The model under review builds one solid part; all positions refer to its coordinate system, in mm. A direction names the side the tool comes from. Give positions to 0.01 mm unless a question says otherwise; leave off trailing zeros. Loops run counter-clockwise (first coordinate to the right, second up) from the corner with the lowest first, then second, coordinate; pieces in that order, holes last. Notation, with made-up numbers: M -40,56.5 L 5,56.5 A15 ccw 5,77.5 Z; hole C 47,31.5 d1. An arc over 180 degrees is marked long. Return JSON: item names as keys, results as strings. Group by question number.
```python
from build123d import *

# Parameters (mm, degrees)
AUFSATZ_LINEAR_AUSTRAGEN1_DEPTH = 18
AUFSATZ_LINEAR_AUSTRAGEN2_DEPTH = 2
SCHNITT_LINEAR_AUSTRAGEN1_REACH = 31.142
SCHNITT_LINEAR_AUSTRAGEN2_REACH = 35.939
SKIZZE5_W                       = 12
SKIZZE5_H                       = 15
SKIZZE7_R                       = 1.22999984
AUFSATZ_LINEAR_AUSTRAGEN3_DEPTH = 6.5
SKIZZE8_R                       = 4.22999984
SKIZZE8_R_2                     = 2.3
AUFSATZ_LINEAR_AUSTRAGEN4_DEPTH = 3
SKIZZE9_W                       = 16.252283896
SKIZZE9_H                       = 8
SKIZZE9_W_2                     = 16.225392475
AUFSATZ_LINEAR_AUSTRAGEN7_DEPTH = 3
SCHNITT_LINEAR_AUSTRAGEN3_REACH = 3.5
SKIZZE11_W                      = 10
SKIZZE11_H                      = 10
SCHNITT_LINEAR_AUSTRAGEN4_REACH = 24.734
SKIZZE13_W                      = 10
SKIZZE13_H                      = 10
SCHNITT_LINEAR_AUSTRAGEN5_REACH = 24.815
SKIZZE14_W                      = 10
SKIZZE14_H                      = 10
SCHNITT_LINEAR_AUSTRAGEN6_REACH = 3.5
SKIZZE15_W                      = 10
SKIZZE15_H                      = 10
SCHNITT_LINEAR_AUSTRAGEN7_REACH = 24.918
SKIZZE16_W                      = 10
SKIZZE16_H                      = 10
SCHNITT_LINEAR_AUSTRAGEN8_REACH = 24.774
SKIZZE17_W                      = 10
SKIZZE17_H                      = 10
SKIZZE18_W                      = 10
SKIZZE18_H                      = 1.5
SCHNITT_LINEAR_AUSTRAGEN9_DEPTH = 8


with BuildPart() as part:
    # Skizze1 → Aufsatz-Linear austragen1 (new body)
    with BuildSketch(Plane.XY):
        Polygon((-22.149859894, 27.765281808), (-11.635793215, 33.83000044), (-10.65000108, 33.83000044), (-10.65000108, 70.94999986), (10.5900012, 70.94999986), (10.5900012, 33.83000044), (11.612735063, 33.83000044), (21.946878227, 27.90320319), (54.822266278, 46.860690996), (65.431940836, 28.488460753), (35.875483821, 11.41999954), (37.79000014, 11.41999954), (37.79000014, -11.66999904), (36.372671479, -11.66999904), (65.402118422, -28.428154068), (54.791716349, -46.801638497), (21.961456264, -27.849347945), (11.636228403, -33.81000048), (10.608764603, -33.81000048), (10.588764643, -70.99999976), (-10.63000112, -70.99999976), (-10.63000112, -33.81000048), (-11.635211495, -33.81000048), (-21.94526311, -27.869445957), (-54.832668225, -46.841377939), (-65.441180026, -28.458395245), (-33.1799992, -9.82193495), (-33.1799992, 9.582671858), (-65.619428736, 28.349034811), (-55.023633975, 46.732102334), align=None)
        Polygon((-22.149950537, 26.033576659), (-11.234189479, 32.33000044), (-9.15000108, 32.33000044), (-9.15000108, 69.44999986), (9.0900012, 69.44999986), (9.0900012, 32.33000044), (11.2131258, 32.33000044), (21.948913697, 26.172853479), (54.272963006, 44.812413555), (63.382848908, 29.03729054), (31.311020441, 10.516235735), (31.653238716, 9.91999954), (36.29000014, 9.91999954), (36.29000014, -10.16999904), (31.252050971, -10.16999904), (31.132619329, -10.37701429), (63.352910716, -28.977183946), (54.242770108, -44.752743199), (21.961450411, -26.11734559), (11.234340849, -32.31000048), (9.109571053, -32.31000048), (9.089571093, -69.49999976), (-9.13000112, -69.49999976), (-9.13000112, -32.31000048), (-11.233987142, -32.31000048), (-21.945708018, -26.138007916), (-54.2831028, -44.792652518), (-63.392584266, -29.007267794), (-31.162137007, -10.388561496), (-31.6799992, -9.546253935), (-31.6799992, 9.963511331), (-31.471105622, 10.326986156), (-63.571974887, 28.897490395), (-54.473438465, 44.682904625), align=None, mode=Mode.SUBTRACT)
    extrude(amount=AUFSATZ_LINEAR_AUSTRAGEN1_DEPTH)

    # Skizze3 → Aufsatz-Linear austragen2 (add)
    with BuildSketch(Plane(origin=(0, 0, 0), x_dir=(-1, 0, 0), z_dir=(0, 0, -1))):
        Polygon((55.023633975, 46.732102334), (22.149859894, 27.765281808), (11.635793215, 33.83000044), (10.65000108, 33.83000044), (10.65000108, 70.94999986), (-10.5900012, 70.94999986), (-10.5900012, 33.83000044), (-11.612735063, 33.83000044), (-21.946878227, 27.90320319), (-54.822266278, 46.860690996), (-65.431940836, 28.488460753), (-35.875483821, 11.41999954), (-37.79000014, 11.41999954), (-37.79000014, -11.66999904), (-36.372671479, -11.66999904), (-65.402118422, -28.428154068), (-54.791716349, -46.801638497), (-21.961456264, -27.849347945), (-11.636228403, -33.81000048), (-10.608764603, -33.81000048), (-10.588764643, -70.99999976), (10.63000112, -70.99999976), (10.63000112, -33.81000048), (11.635211495, -33.81000048), (21.94526311, -27.869445957), (54.832668225, -46.841377939), (65.441180026, -28.458395245), (33.1799992, -9.82193495), (33.1799992, 9.582671858), (65.619428736, 28.349034811), align=None)
    extrude(amount=AUFSATZ_LINEAR_AUSTRAGEN2_DEPTH)

    # Skizze4 → Schnitt-Linear austragen1 (cut, up to next)
    with BuildSketch(Plane.ZY.offset(-36.29000014), mode=Mode.PRIVATE) as schnitt_linear_austragen1_sk1:
        Polygon((17.00382914, 9.91999954), (17.00382914, -10.16999904), (0.851260669, -10.16999904), (0, -10.16999904), (0, 9.91999954), (0.851260669, 9.91999954), align=None)
    schnitt_linear_austragen1_tool1 = extrude(schnitt_linear_austragen1_sk1.sketch, amount=-SCHNITT_LINEAR_AUSTRAGEN1_REACH, mode=Mode.PRIVATE) & part.part
    add(schnitt_linear_austragen1_tool1.solids().sort_by_distance((36.29, -0.125, 8.501915))[0], mode=Mode.SUBTRACT)

    # Skizze5 → Schnitt-Linear austragen2 (cut, up to next)
    with BuildSketch(Plane(origin=(-31.6799992, 0, 0), x_dir=(0, 0, -1), z_dir=(1, 0, 0)), mode=Mode.PRIVATE) as schnitt_linear_austragen2_sk1:
        with Locations((-6, 0)):
            Rectangle(SKIZZE5_W, SKIZZE5_H)
    schnitt_linear_austragen2_tool1 = extrude(schnitt_linear_austragen2_sk1.sketch, amount=-SCHNITT_LINEAR_AUSTRAGEN2_REACH, mode=Mode.PRIVATE) & part.part
    add(schnitt_linear_austragen2_tool1.solids().sort_by_distance((-31.679999, 0, 6))[0], mode=Mode.SUBTRACT)

    # Skizze7 → Aufsatz-Linear austragen3 (add)
    with BuildSketch(Plane.XY):
        with Locations((0, 15.00000048)):
            Circle(SKIZZE7_R)
        with Locations((0, -18.5000011)):
            Circle(SKIZZE7_R)
        with Locations((-9.1899994, -20.2700001)):
            Circle(SKIZZE7_R)
    extrude(amount=AUFSATZ_LINEAR_AUSTRAGEN3_DEPTH)

    # Skizze8 → Aufsatz-Linear austragen4 (add)
    with BuildSketch(Plane.XY):
        with Locations((-9.1899994, -20.2700001)):
            Circle(SKIZZE8_R)
        with Locations((0, -18.5000011)):
            Circle(SKIZZE8_R)
        with Locations((13.9, 25.897140228)):
            Circle(SKIZZE8_R_2)
        with Locations((-13.9, 25.897140228)):
            Circle(SKIZZE8_R_2)
        with Locations((13.9, -24.8615628)):
            Circle(SKIZZE8_R_2)
        with Locations((-13.9, -24.8615628)):
            Circle(SKIZZE8_R_2)
        with BuildLine():
            Line((3.936452455, 16.548303007), (-3.936452455, 16.548303007))
            ThreePointArc((-3.936452455, 16.548303007), (0, 10.77000064), (3.936452455, 16.548303007))
        make_face()
    extrude(amount=AUFSATZ_LINEAR_AUSTRAGEN4_DEPTH)

    # Skizze9 → Aufsatz-Linear austragen7 (add)
    with BuildSketch(Plane.XY):
        Polygon((-39.106966425, 34.662574989), (-47.255864546, 20.538698219), (-40.326487672, 16.540731718), (-32.177589551, 30.664608488), align=None)
        with Locations((-0.036140748, 47.33000044)):
            Rectangle(SKIZZE9_W, SKIZZE9_H)
        Polygon((40.096213315, 16.744336658), (31.986065924, 30.788205039), (38.913859811, 34.78891396), (47.024007202, 20.745045579), align=None)
        Polygon((40.10078632, -16.697308213), (47.029196881, -20.696949084), (38.916380603, -34.750441337), (31.987970041, -30.750800466), align=None)
        with Locations((-0.017304883, -47.31000048)):
            Rectangle(SKIZZE9_W_2, SKIZZE9_H)
        Polygon((-38.906027405, -34.762365837), (-31.978796823, -30.760681634), (-40.098111463, -16.705508406), (-47.025342045, -20.70719261), align=None)
    extrude(amount=AUFSATZ_LINEAR_AUSTRAGEN7_DEPTH)

    # Skizze11 → Schnitt-Linear austragen3 (cut, up to next)
    with BuildSketch(Plane.XZ.offset(-69.44999986), mode=Mode.PRIVATE) as schnitt_linear_austragen3_sk1:
        with Locations((0, 5)):
            Rectangle(SKIZZE11_W, SKIZZE11_H)
    schnitt_linear_austragen3_tool1 = extrude(schnitt_linear_austragen3_sk1.sketch, amount=-SCHNITT_LINEAR_AUSTRAGEN3_REACH, mode=Mode.PRIVATE) & part.part
    add(schnitt_linear_austragen3_tool1.solids().sort_by_distance((0, 69.45, 5))[0], mode=Mode.SUBTRACT)

    # Skizze13 → Schnitt-Linear austragen4 (cut, up to next)
    with BuildSketch(Plane(origin=(60.106593545, 34.710614216, 0), x_dir=(0, 0, 1), z_dir=(-0.86597514, -0.500087049, 0)), mode=Mode.PRIVATE) as schnitt_linear_austragen4_sk1:
        with Locations((5, 2.556930019)):
            Rectangle(SKIZZE13_W, SKIZZE13_H)
    schnitt_linear_austragen4_tool1 = extrude(schnitt_linear_austragen4_sk1.sketch, amount=-SCHNITT_LINEAR_AUSTRAGEN4_REACH, mode=Mode.PRIVATE) & part.part
    add(schnitt_linear_austragen4_tool1.solids().sort_by_distance((58.827906, 36.924852, 5))[0], mode=Mode.SUBTRACT)

    # Skizze14 → Schnitt-Linear austragen5 (cut, up to next)
    with BuildSketch(Plane(origin=(60.058107222, -34.682624727, 0), x_dir=(0, 0, 1), z_dir=(-0.865975074, 0.500087164, 0)), mode=Mode.PRIVATE) as schnitt_linear_austragen5_sk1:
        with Locations((5, -2.520094297)):
            Rectangle(SKIZZE14_W, SKIZZE14_H)
    schnitt_linear_austragen5_tool1 = extrude(schnitt_linear_austragen5_sk1.sketch, amount=-SCHNITT_LINEAR_AUSTRAGEN5_REACH, mode=Mode.PRIVATE) & part.part
    add(schnitt_linear_austragen5_tool1.solids().sort_by_distance((58.79784, -36.864964, 5))[0], mode=Mode.SUBTRACT)

    # Skizze15 → Schnitt-Linear austragen6 (cut, up to next)
    with BuildSketch(Plane(origin=(0, -69.49999976, 0), x_dir=(1, 0, 0), z_dir=(0, 1, 0)), mode=Mode.PRIVATE) as schnitt_linear_austragen6_sk1:
        with Locations((-0.020215013, -5)):
            Rectangle(SKIZZE15_W, SKIZZE15_H)
    schnitt_linear_austragen6_tool1 = extrude(schnitt_linear_austragen6_sk1.sketch, amount=-SCHNITT_LINEAR_AUSTRAGEN6_REACH, mode=Mode.PRIVATE) & part.part
    add(schnitt_linear_austragen6_tool1.solids().sort_by_distance((-0.020215, -69.5, 5))[0], mode=Mode.SUBTRACT)

    # Skizze16 → Schnitt-Linear austragen7 (cut, up to next)
    with BuildSketch(Plane(origin=(-60.113041463, -34.690230655, 0), x_dir=(0, 0, -1), z_dir=(0.866125522, 0.49982655, 0)), mode=Mode.PRIVATE) as schnitt_linear_austragen7_sk1:
        with Locations((-5, -2.551280899)):
            Rectangle(SKIZZE16_W, SKIZZE16_H)
    schnitt_linear_austragen7_tool1 = extrude(schnitt_linear_austragen7_sk1.sketch, amount=-SCHNITT_LINEAR_AUSTRAGEN7_REACH, mode=Mode.PRIVATE) & part.part
    add(schnitt_linear_austragen7_tool1.solids().sort_by_distance((-58.837844, -36.89996, 5))[0], mode=Mode.SUBTRACT)

    # Skizze17 → Schnitt-Linear austragen8 (cut, up to next)
    with BuildSketch(Plane(origin=(-60.221224503, 34.710841064, 0), x_dir=(0, 0, -1), z_dir=(0.866385869, -0.499375136, 0)), mode=Mode.PRIVATE) as schnitt_linear_austragen8_sk1:
        with Locations((-5, 2.400035044)):
            Rectangle(SKIZZE17_W, SKIZZE17_H)
    schnitt_linear_austragen8_tool1 = extrude(schnitt_linear_austragen8_sk1.sketch, amount=-SCHNITT_LINEAR_AUSTRAGEN8_REACH, mode=Mode.PRIVATE) & part.part
    add(schnitt_linear_austragen8_tool1.solids().sort_by_distance((-59.022707, 36.790198, 5))[0], mode=Mode.SUBTRACT)

    # Skizze18 → Schnitt-Linear austragen9 (cut)
    with BuildSketch(Plane(origin=(0, 0, 10), x_dir=(-1, 0, 0), z_dir=(0, 0, -1))):
        Polygon((-62.597238843, -33.285218949), (-57.596367204, -41.944969687), (-56.297404593, -41.194838941), (-61.298276232, -32.535088203), align=None)
        with Locations((0.020215013, -70.24999976)):
            Rectangle(SKIZZE18_W, SKIZZE18_H)
        Polygon((57.637899065, -41.980327591), (62.636164566, -33.319072372), (61.336976284, -32.569332546), (56.338710782, -41.230587766), align=None)
        Polygon((62.81916116, 33.207330871), (57.825409798, 41.871189557), (56.525830995, 41.122126853), (61.519582357, 32.458268167), align=None)
        with Locations((0, 70.19999986)):
            Rectangle(SKIZZE18_W, SKIZZE18_H)
        Polygon((-57.626433421, 42.004858322), (-62.627303913, 33.345106921), (-61.328341203, 32.594976347), (-56.327470711, 41.254727748), align=None)
    extrude(amount=-SCHNITT_LINEAR_AUSTRAGEN9_DEPTH, mode=Mode.SUBTRACT)


solid = part.part
```
(1) For faces 4 (the flat face through (38.154, 37.249, 8.14)), 5 (the flat face through (37, 0, 18)), 6 (the cylindrical face through (12.075, -26.261, 1.479)), 7 (the flat face through (50.861, 20.074, 8.14)), list the 3-axis set-ups (+Z, -Z, +X, -X, +Y, -Y) from which the entire face can be reached by the end or side of a thin tool; tool diameter is ignored.
(2) Add section A-A (x = -35). Write out the cut boundary in (y, z), and give its area (3 significant figures).
(3) For pin 1 (0.7 mm diameter, centred on x = 0, y = 14.5, fed in from +Z); pin 2 (5.5 mm diameter, centred on y = -51.5, z = 6, fed in from +X); pin 3 (8 mm diameter, centred on x = 26.5, z = 7, fed in from -Y), all flat-tipped, find the tip position at first contact; note any pin that passes through.
(4) Mouldability with a two-part tool opening along Y and no side actions: class faces 1 (the flat face through (44, 19, 1)), 2 (the flat face through (10.59, 53, 8)), 3 (the flat face through (63.59, 31.68, 8.14)) as released by +Y, released by -Y, zero draft, split by the parting line, or undercut.
(5) Add section B-B (x = 13.9). Write out the cut boundary in (y, z).
(6) For probe 1 along X at (y, z) = (-54, 12.5); probe 2 along Y at (x, z) = (6, 5.75); probe 3 along Y at (x, z) = (46, 6.5), list the stretches that pass through material, from the lowest coordinate up.
Verdict:
{
 "1": {"face 4": "+Z, -Z, +Y", "face 5": "+Z, +X, -X, +Y, -Y", "face 6": "+Z", "face 7": "+Z, -Z, +X"},
 "2": {"outline": "M -35.4,-2 L -10.87,-2 L -10.87,18 L -12.61,18 L -12.61,0 L -25.53,0 L -25.53,3 L -32.51,3 L -32.51,0 L -33.67,0 L -33.67,18 L -35.4,18 Z; M 10.64,-2 L 35.18,-2 L 35.18,18 L 33.45,18 L 33.45,0 L 32.29,0 L 32.29,3 L 25.77,3 L 25.77,0 L 12.37,0 L 12.37,18 L 10.64,18 Z", "area": "263 mm²"},
 "3": {"pin 1": "stops at z = 6.5", "pin 2": "stops at x = 10.6", "pin 3": "stops at y = -32.78"},
 "4": {"face 1": "undercut", "face 2": "zero draft", "face 3": "released by +Y"},
 "5": {"outline": "M -32.5,-2 L 32.52,-2 L 32.52,18 L 30.79,18 L 30.79,0 L 28.2,0 L 28.2,3 L 23.6,3 L 23.6,0 L -22.56,0 L -22.56,3 L -27.16,3 L -27.16,0 L -30.77,0 L -30.77,18 L -32.5,18 Z"},
 "6": {"probe 1": "x = -10.63 to -9.13, 9.1 to 10.6", "probe 2": "y = -71 to -69.5, 69.45 to 70.95", "probe 3": "y = -41.73 to -39.99, -18.96 to -17.23, 17.27 to 19, 40.04 to 41.77"}
}
